Could you check a few things on this model? Use its own coordinates, in mm. A direction names the side the tool comes from. Give positions to 0.01 mm unless a question says otherwise; leave off trailing zeros. Order: outer loops, then holes, each group sorted by start corner. A loop starts at its lowest first (then second) coordinate and runs counter-clockwise, first axis right, second up. Notation, with made-up numbers: (20, 12) - (58, 12) arc R16 ccw to (58, 31) - close; hole circle Ø10 at (-13.5, 27.25). An arc over 180 degrees is marked (long way). One line per question, with ' | ' between items. Start each with the question number.
1. If we mould it in two halves opening along Y, with no side actions, what happens to faces 1 (the cylindrical face through (10.07, -6.834, 17.3)), 2 (the flat face through (10, 10, 0)), 3 (the cylindrical face through (10, -3, 14))? For each: released by +Y, released by -Y, zero draft, split by the parting line, or undercut.
2. Imagine slicing it at B-B (z = 12.5). Please give me the cut outline in (x, y), and give its area (3 significant figures).
3. Imagine slicing it at D-D (x = 4.25). Please give me the cut outline in (y, z).
4. Which directions (+Z, -Z, +X, -X, +Y, -Y) give clear straight access to the entire face, cutting with the end or side of a thin tool? Please do faces 4 (the flat face through (5, -2, 15)), 5 (the flat face through (10, 0, 6)), 6 (the flat face through (15, -2, 15)), 7 (the flat face through (20, 10, 5)), 8 (the flat face through (10, 20, 5)).
5. Imagine slicing it at A-A (x = 11.5). Please give me the cut outline in (y, z), and give its area (3 significant figures).
6. For P1, Ø4, axis at x = 13, z = 17, coming from the -Y side; P2, Ø2, axis at y = -6.5, z = 4.5, coming from the -X side; P3, Ø4, axis at y = 6.5, z = 17.5, coming from the +X side, each with a flat end and sliding along its axis, tell me the tip position at first contact or that it passes through.
7. I need wall thicknesses on probe 1 along Y at (x, z) = (1.25, 1); probe 2 along X at (y, z) = (-6, 3.5); probe 3 along Z at (x, y) = (11.75, 3.75). Which ranges of each line are inside material? Lowest first, please. Write a range as from..to.
8. Imagine slicing it at C-C (y = -4.25). Please give me the cut outline in (x, z), and give its area (3 significant figures).
```python
from build123d import *

# Parameters (mm, degrees)
SKETCH_1_W    = 20
SKETCH_1_H    = 20
BASEBOX_DEPTH = 10
SKETCH_2_W    = 10
SKETCH_2_H    = 5


with BuildPart() as part:
    # 草图1 → BaseBox (new body)
    with BuildSketch(Plane.XY):
        with Locations((10, 10)):
            Rectangle(SKETCH_1_W, SKETCH_1_H)
    extrude(amount=BASEBOX_DEPTH)

    # 草图2 → RevolveAxisEdge (revolve)
    with BuildSketch(Plane.XY.offset(10)):
        with Locations((10, 7.5)):
            Rectangle(SKETCH_2_W, SKETCH_2_H)
    revolve(axis=Axis((0, 0, 10), (1, 0, 0)))


solid = part.part
```
Results found:
1) face 1: split by the parting line | face 2: zero draft | face 3: undercut
2) outline: (5, -9.68) - (15, -9.68) - (15, -4.33) - (5, -4.33) - close; (5, 4.33) - (15, 4.33) - (15, 9.68) - (5, 9.68) - close | area: 107 mm2
3) outline: (0, 0) - (20, 0) - (20, 10) - (0, 10) - close
4) face 4: +Z, -X, -Y | face 5: none | face 6: +Z, +X, -Y | face 7: +Z, -Z, +X, +Y, -Y | face 8: +Z, -Z, +X, -X, +Y
5) outline: (0, 0) - (20, 0) - (20, 10) - (10, 10) arc R10 ccw (long way) to start; hole (0, 5) - (0, 10) - (5, 10) arc R5 ccw (long way) to start | area: 377 mm2
6) P1: stops at y = -8.66 | P2: stops at x = 5 | P3: stops at x = 15
7) probe 1: y = 0..20 | probe 2: x = 5..15 | probe 3: z = 0..10, 13.31..19.27
8) outline: (5, 0.95) - (15, 0.95) - (15, 7.37) - (5, 7.37) - close; (5, 12.63) - (15, 12.63) - (15, 19.05) - (5, 19.05) - close | area: 128 mm2
